Autodesk Inventor part; units mm, degrees
ref_plane "YZ Plane" through (0, 0, 0) normal (1, 0, 0) x (0, 1, 0)
ref_plane "XZ Plane" through (0, 0, 0) normal (0, 1, 0) x (-1, 0, 0)
ref_plane "XY Plane" through (0, 0, 0) normal (0, 0, 1) x (1, 0, 0)
sketch "スケッチ1" plane through (0, 0, 0) normal (0, 0, 1) x (1, 0, 0)
  line L0 (18, 0) -> (18, 200)
  line L1 (0, 200) -> (0, 0)
  line L2 (9, 200) -> (9, 0) construction
  arc A0 (18, 200) -> (0, 200) centre (9, 200) ccw
  arc A1 (0, 0) -> (18, 0) centre (9, 0) ccw
  circle A2 centre (9, 0) radius 3.5
  circle A3 centre (9, 200) radius 3.5
  dimension "d35" = 18
  dimension "d36" = 200
  dimension "d37" = 7
  dimension "d38" = 7
extrude "押し出し1" add sketch "スケッチ1" along normal blind 2
properties part number "foot_link" material "GFRP"
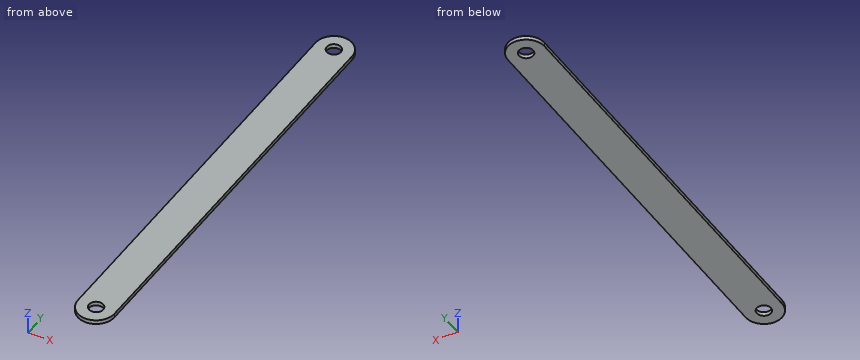
Geometry: final body of the model. Coordinates: model frame, mm. Give positions to 0.01 mm unless a question says otherwise; leave off trailing zeros. Loops run counter-clockwise (first coordinate to the right, second up) from the corner with the lowest first, then second, coordinate; pieces in that order, holes last. Notation, with made-up numbers: M 17,-14.5 L 26,-14.5 A21 ccw 26,-7.5 Z; hole C -39.5,11.5 d8. An arc over 180 degrees is marked long. Put each result on its own line as item: value.
1) Material intervals for L1, parallel to Y at x = 9, z = 1.1; L2, parallel to Y at x = 11.75, z = 1.8; L3, parallel to Y at x = 17, z = 1.9, sorted ascending. Write a range as from..to.
Computed values:
L1: y = -9..-3.5, 3.5..196.5, 203.5..209
L2: y = -8.57..-2.17, 2.17..197.83, 202.17..208.57
L3: y = -4.12..204.12
2) Cut plane A-A, the plane x = 9. Return the cut outline in (y, z), plus the area to 3 significant figures.
Computed values:
outline: M -9,0 L -3.5,0 L -3.5,2 L -9,2 Z; M 3.5,0 L 196.5,0 L 196.5,2 L 3.5,2 Z; M 203.5,0 L 209,0 L 209,2 L 203.5,2 Z
area: 408 mm^2
3) Cut plane B-B, the plane z = 1.4. Return the cut outline in (x, y), plus the area to 3 significant figures.
Computed values:
outline: M 0,0 A9 ccw 18,0 L 18,200 A9 ccw 0,200 Z; hole C 9,0 d7; hole C 9,200 d7
area: 3,780 mm^2
